Geometry check sheet. Reference: the model listing, model coordinates, mm. Face numbers are marked on the shaded views. A direction names the side the tool comes from. Coordinates: 2 decimals unless noted, no trailing zeros. Loops run counter-clockwise (first coordinate to the right, second up) from the corner with the lowest first, then second, coordinate; pieces in that order, holes last.
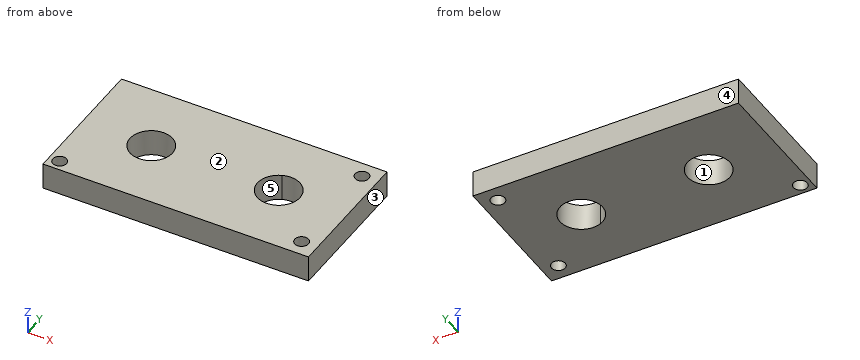
Autodesk Inventor part; units mm, degrees
ref_plane "YZ Plane" through (0, 0, 0) normal (1, 0, 0) x (0, 1, 0)
ref_plane "XZ Plane" through (0, 0, 0) normal (0, 1, 0) x (-1, 0, 0)
ref_plane "XY Plane" through (0, 0, 0) normal (0, 0, 1) x (1, 0, 0)
sketch "Sketch1" plane through (0, 0, 0) normal (0, 0, 1) x (1, 0, 0)
  line L0 (0, 0) -> (58.42, 0)
  line L1 (58.42, 0) -> (58.42, -33.02)
  line L2 (58.42, -33.02) -> (0, -33.02)
  line L3 (0, -33.02) -> (0, 0)
  dimension "d0" = 58.42
  dimension "d1" = 33.02
extrude "Extrusion1" add sketch "Sketch1" along normal blind 6.35
sketch "Sketch4" plane through (0, 0, 6.35) normal (0, 0, 1) x (1, 0, 0)
  point P0 (0, 0)
sketch "Sketch5" plane through (58.42, -33.02, 0) normal (1, 0, 0) x (0, 0, -1)
  line L0 (-6.35, 33.02) -> (-6.35, 0)
  line L1 (0, 33.02) -> (-6.35, 33.02)
  line L2 (-6.35, 33.02) -> (-6.35, 0)
  line L3 (-6.35, 0) -> (0, 0)
  line L4 (0, 0) -> (0, 33.02)
extrude "Extrusion4" add sketch "Sketch5" along normal blind 5.08
sketch "Sketch6" plane through (0, 0, 6.35) normal (0, 0, 1) x (1, 0, 0)
  circle A0 centre (15.24, -16.51) radius 5.08
  line L0 (0, 0) -> (63.5, 0)
  line L1 (0, 0) -> (0, -33.02)
  circle A1 centre (41.91, -16.51) radius 5.08
  dimension "d16" = 10.16
  dimension "d17" = 16.51
  dimension "d18" = 15.24
  dimension "d19" = 10.16
  dimension "d20" = 26.67
extrude "Extrusion5" cut sketch "Sketch6" against normal blind 7.62
sketch "Sketch7" plane through (0, -33.02, 0) normal (-1, 0, 0) x (0, 0, 1)
  line L0 (6.35, 33.02) -> (6.35, 0)
  line L1 (0, 33.02) -> (6.35, 33.02)
  line L2 (6.35, 33.02) -> (6.35, 0)
  line L3 (6.35, 0) -> (0, 0)
  line L4 (0, 0) -> (0, 33.02)
extrude "Extrusion6" add sketch "Sketch7" along normal blind 2.54
sketch "Sketch8" plane through (-2.54, -33.02, 0) normal (-1, 0, 0) x (0, 0, 1)
  line L0 (6.35, 0) -> (0, 0)
  line L1 (0, 33.02) -> (6.35, 33.02)
  line L2 (6.35, 33.02) -> (6.35, 0)
  line L3 (6.35, 0) -> (0, 0)
  line L4 (0, 0) -> (0, 33.02)
extrude "Extrusion7" cut sketch "Sketch8" against normal blind 1.27
sketch "Sketch10" plane through (63.5, -33.02, 0) normal (1, 0, 0) x (0, 0, -1)
  line L0 (0, 33.02) -> (-6.35, 33.02)
  line L1 (-6.35, 33.02) -> (0, 33.02)
  line L2 (0, 33.02) -> (0, 0)
  line L3 (0, 0) -> (-6.35, 0)
  line L4 (-6.35, 0) -> (-6.35, 33.02)
extrude "Extrusion9" cut sketch "Sketch10" against normal blind 1.27
sketch "Sketch11" plane through (0, 0, 6.35) normal (0, 0, 1) x (1, 0, 0)
  circle A0 centre (58.42, -3.81) radius 1.651
  circle A1 centre (58.42, -29.21) radius 1.651
  line L0 (62.23, -33.02) -> (62.23, 0)
  line L1 (-1.27, 0) -> (62.23, 0)
  line L2 (62.23, -33.02) -> (-1.27, -33.02)
  point P0 (0, 0)
  dimension "d37" = 3.302
  dimension "d38" = 3.302
  dimension "d39" = 3.81
  dimension "d40" = 3.81
  dimension "d41" = 3.81
  dimension "d42" = 3.81
extrude "Extrusion10" cut sketch "Sketch11" against normal blind 6.35
sketch "Sketch12" plane through (0, 0, 6.35) normal (0, 0, 1) x (1, 0, 0)
  circle A0 centre (1.27, -30.48) radius 1.651
  line L0 (62.23, -33.02) -> (-1.27, -33.02)
  line L1 (-1.27, 0) -> (-1.27, -33.02)
  point P0 (0, 0)
  dimension "d45" = 3.302
  dimension "d46" = 2.54
  dimension "d47" = 2.54
extrude "Extrusion11" cut sketch "Sketch12" against normal blind 6.35
sketch "Sketch14" plane through (0, 0, 6.35) normal (0, 0, 1) x (1, 0, 0)
  line L0 (62.23, -33.02) -> (-1.27, -33.02)
  circle A0 centre (15.24, -16.51) radius 5.08
  circle A1 centre (45.72, -16.51) radius 5.08
  circle A2 centre (45.72, -16.51) radius 9.5628
  point P0 (0, 0)
  dimension "d55" = 16.51
  dimension "d56" = 30.48
  dimension "d57" = 10.16
extrude "Extrusion13" add sketch "Sketch14" against normal blind 25.4 contours A2
sketch "Sketch15" plane through (0, 0, 6.35) normal (0, 0, 1) x (1, 0, 0)
  arc A0 (43.815, -21.2193) -> (43.815, -11.8007) centre (45.72, -16.51) ccw
  circle A1 centre (45.72, -16.51) radius 5.08
  point P0 (0, 0)
  dimension "d60" = 10.16
extrude "Extrusion14" cut sketch "Sketch15" against normal blind 25.4
sketch "Sketch16" plane through (62.23, -33.02, 0) normal (1, 0, 0) x (0, 0, -1)
  line L0 (0, 33.02) -> (24.9561, 33.02)
  line L1 (24.9561, 33.02) -> (24.9561, -0.1066)
  line L2 (24.9561, -0.1066) -> (0, -0.1066)
  line L3 (0, -0.1066) -> (0, 33.02)
extrude "Extrusion15" cut sketch "Sketch16" against normal blind 50.8
properties part number "claw attachment back"
1) Section check C-C on x = 45.72. Record the cut outline in (y, z), and give its area (3 significant figures).
Data:
outline: (-33.02, 0) - (-21.59, 0) - (-21.59, 6.35) - (-33.02, 6.35) - close; (-11.43, 0) - (0, 0) - (0, 6.35) - (-11.43, 6.35) - close
area: 145 mm2
2) Mould release check, pull along X, two halves, no side actions. Record for the marked faces 1, 2 and 3: +X half, -X half, draft (parallel to the pull), parting line (faces both ways), or undercut.
Data:
face 1: undercut
face 2: draft
face 3: +X half
3) Section check B-B on x = 58.42. Record the cut outline in (y, z), and give its area (3 significant figures).
Data:
outline: (-33.02, 0) - (-30.86, 0) - (-30.86, 6.35) - (-33.02, 6.35) - close; (-27.56, 0) - (-5.46, 0) - (-5.46, 6.35) - (-27.56, 6.35) - close; (-2.16, 0) - (0, 0) - (0, 6.35) - (-2.16, 6.35) - close
area: 168 mm2
4) Material ranges on probe 1 along X at (y, z) = (-16.51, 2); probe 2 along Y at (x, z) = (58.42, 2); probe 3 along Y at (x, z) = (15.24, 4), recorded low to high.
Data:
probe 1: x = -1.27 to 10.16, 20.32 to 40.64, 50.8 to 62.23
probe 2: y = -33.02 to -30.86, -27.56 to -5.46, -2.16 to 0
probe 3: y = -33.02 to -21.59, -11.43 to 0
5) Access from +Z, -Z, +X, -X, +Y, -Y to the whole of each face (thin tool, end or side, straight path). Record for the marked faces 4 and 5.
Data:
face 4: +Z, -Z, +X, -X, +Y
face 5: +Z, -Z
6) Section check A-A on y = -16.51. Record the cut outline in (x, z).
Data:
outline: (-1.27, 0) - (10.16, 0) - (10.16, 6.35) - (-1.27, 6.35) - close; (20.32, 0) - (40.64, 0) - (40.64, 6.35) - (20.32, 6.35) - close; (50.8, 0) - (62.23, 0) - (62.23, 6.35) - (50.8, 6.35) - close
7) Section check D-D on z = 2.5. Record the cut outline in (x, y) (3 decimals).
Data:
outline: (-1.27, -33.02) - (62.23, -33.02) - (62.23, 0) - (-1.27, 0) - close; hole circle Ø3.302 at (1.27, -30.48); hole circle Ø10.16 at (15.24, -16.51); hole (43.815, -21.219) arc R5.08 ccw (long way) to (43.815, -11.801) arc R5.08 ccw to start; hole circle Ø3.302 at (58.42, -29.21); hole circle Ø3.302 at (58.42, -3.81)
